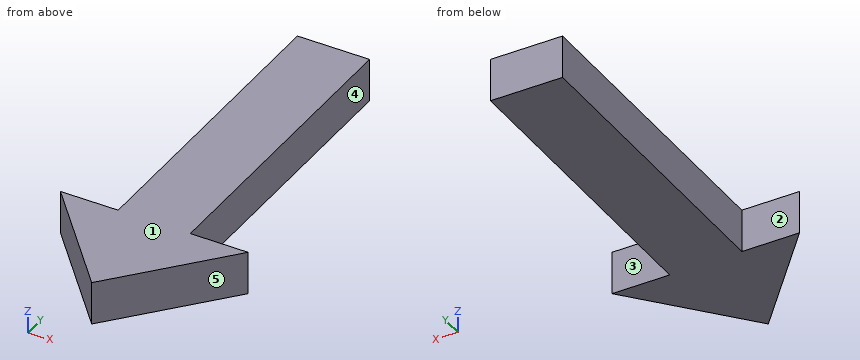
```python
from build123d import *

# Parameters (mm, degrees)
F0_W     = 12.7
F0_H     = 7.62
F1_DEPTH = 63.5
F4_DEPTH = 7.62


with BuildPart() as f1:
    # F0 (on Front) → F1 (new body)
    with BuildSketch(Plane.XZ):
        with Locations((6.35, -3.81)):
            Rectangle(F0_W, F0_H)
    extrude(amount=F1_DEPTH)

    # F3 (on face) → F4 (join)
    with BuildSketch(Plane.XY):
        Polygon((22.86, -54.61), (-10.16, -54.61), (6.35, -73.66), align=None)
    extrude(amount=-F4_DEPTH)


solid = f1.part
```
Check sheet for the modelled part. Datum: model origin and axes. Units: mm. Face numbers are marked on the shaded views. A direction names the side the tool comes from. Give positions to 0.01 mm unless a question says otherwise; leave off trailing zeros. Order: outer loops, then holes, each group sorted by start corner. A loop starts at its lowest first (then second) coordinate and runs counter-clockwise, first axis right, second up. Notation, with made-up numbers: (42.25, 38) -> (95.25, 38) arc R13 cw to (95.25, 61) -> close; hole circle Ø8 at (89.5, -17). An arc over 180 degrees is marked (long way). Use CSV: the item, a comma, the result in double quotes. Start each with the question number.
1) Set-up check for the marked faces 1 and 2: record each of +Z, -Z, +X, -X, +Y, -Y from which the full face is reachable in a straight line by a thin tool's end or side.
2) Material ranges on line 1 (X direction, y = -49, z = -0.5); line 2 (Y direction, x = -1.5, z = -5.5); line 3 (Y direction, x = 9.5, z = -3.5), recorded low to high. Write a range as from..to.
3) Sectioned sample at A-A, the plane z = -3. Record the boundary of the cut face in (x, y), plus the area to 3 significant figures.
4) Sectioned sample at B-B, the plane x = -6. Record the boundary of the cut face in (y, z), plus the area to 3 significant figures.
5) Sectioned sample at C-C, the plane y = -36. Record the boundary of the cut face in (x, z).
6) Mould release check, pull along Y, two halves, no side actions. Record for the marked faces 3, 4 and 5: released by +Y, released by -Y, zero draft, split by the parting line, or undercut.
7) Go/stop test with flat-tipped pins: P1, Ø4, axis at y = -64.5, z = -5, coming from the +X side; P2, Ø2.5, axis at y = -22, z = -5.5, coming from the +X side; P3, Ø1.5, axis at x = 8, z = -1.5, coming from the -Y side. Record where each tip stops, or that it passes through.
Recorded:
1,face 1,"+Z, +X, -X, +Y, -Y"
1,face 2,"+Z, -Z, -X, +Y"
2,line 1,"0..12.7"
2,line 2,"-64.6..-54.61"
2,line 3,"-70.03..0"
3,outline,"(-10.16, -54.61) -> (6.35, -73.66) -> (22.86, -54.61) -> (12.7, -54.61) -> (12.7, 0) -> (0, 0) -> (0, -54.61) -> close"
3,area,"1,010 mm2"
4,outline,"(-59.41, -7.62) -> (-54.61, -7.62) -> (-54.61, 0) -> (-59.41, 0) -> close"
4,area,"36.6 mm2"
5,outline,"(0, -7.62) -> (12.7, -7.62) -> (12.7, 0) -> (0, 0) -> close"
6,face 3,"released by +Y"
6,face 4,"zero draft"
6,face 5,"released by -Y"
7,P1,"x = 16.02"
7,P2,"x = 12.7"
7,P3,"y = -72.62"
